The listing builds one solid part. Answer for the finished solid, in the listing's coordinates (mm). A direction names the side the tool comes from. Round coordinates to 2 decimals unless told otherwise and drop trailing zeros. Order: outer loops, then holes, each group sorted by start corner. A loop starts at its lowest first (then second) coordinate and runs counter-clockwise, first axis right, second up. Notation, with made-up numbers: (16.25, -28.5) - (60.25, -28.5) arc R23 ccw to (60.25, -19.5) - close; hole circle Ø2 at (-14.5, -4). An arc over 180 degrees is marked (long way). Write item = value, one per line.
from build123d import *

# Parameters (mm, degrees)
F0_R           = 31.75
F0_R_2         = 15.875
F1_DEPTH       = 50.8
F2_R           = 9.525
F3_DEPTH       = 31.75
F5_D           = 19.05
F5_CSINK_D     = 31.75
F5_CSINK_ANGLE = 82
F7_DEPTH       = 76.2


with BuildPart() as f1:
    # F0 (on Front) → F1 (new body)
    with BuildSketch(Plane.XZ):
        Circle(F0_R)
        Circle(F0_R_2, mode=Mode.SUBTRACT)
    extrude(amount=F1_DEPTH)

    # F2 (on Front) → F3 (join)
    with BuildSketch(Plane.XZ):
        with BuildLine():
            Line((76.2, 25.49937), (18.47559, 25.49937))
            Line((18.47559, 25.49937), (18.47559, -25.30063))
            Line((18.47559, -25.30063), (76.2, -25.30063))
            ThreePointArc((76.2, -25.30063), (101.6, 0.09937), (76.2, 25.49937))
        make_face()
        with Locations((76.2, 0)):
            Circle(F2_R, mode=Mode.SUBTRACT)
    extrude(amount=F3_DEPTH)

    # F5 (through all)
    with Locations(Plane.XZ.offset(31.75)):
        with Locations((76.2, 0.09937)):
            CounterSinkHole(F5_D / 2, F5_CSINK_D / 2, counter_sink_angle=F5_CSINK_ANGLE)

    # F6 (on face) → F7 (cut)
    with BuildSketch(Plane.XZ.offset(50.8)):
        with BuildLine():
            ThreePointArc((15.875, 0), (15.691131, -2.409153), (15.143785, -4.7625))
            Line((15.143785, -4.7625), (19.906285, -4.7625))
            Line((19.906285, -4.7625), (19.906285, 4.7625))
            Line((19.906285, 4.7625), (15.143785, 4.7625))
            ThreePointArc((15.143785, 4.7625), (15.691131, 2.409153), (15.875, 0))
        make_face()
    extrude(amount=-F7_DEPTH, mode=Mode.SUBTRACT)


solid = f1.part
Q1. Section A-A on x = 0 is taken. Determine the outline of the cut face in (y, z) (3 decimals).
Model answer:
outline = (-50.8, -31.75) - (0, -31.75) - (0, -15.875) - (-50.8, -15.875) - close; (-50.8, 15.875) - (0, 15.875) - (0, 31.75) - (-50.8, 31.75) - close
Q2. Determine the mould class of faces 4 (the face through (47, -16, -25.301)), 5 (the face through (101.594, -15.653, -0.459)), 6 (the face through (-15.862, -25.044, 0.63)) for opening direction Z: released by +Z, released by -Z, zero draft, split by the parting line, or undercut.
Model answer:
face_4 = released by -Z
face_5 = split by the parting line
face_6 = undercut
Q3. For faces 1 (the face through (34, 0, 0)), 2 (the face through (48, -16, 25.499)), 3 (the face through (75.99, -12.051, 9.622)), determine the directions among +Z, -Z, +X, -X, +Y, -Y from which every point of the face is accessible in a straight line to the end or side of a thin tool.
Model answer:
face_1 = +Z, -Z, +X, -X, +Y
face_2 = +Z, +X, +Y, -Y
face_3 = +Y, -Y
Q4. Section D-D on z = 18 is taken. Determine the outline of the cut face in (x, y).
Model answer:
outline = (-26.15, -50.8) - (26.15, -50.8) - (26.15, -31.75) - (94.22, -31.75) - (94.22, 0) - (-26.15, 0) - close
Q5. Flat-ended cylindrical pins translate along their axes: P1, Ø9.5, axis at x = 49.5, y = -15.5, coming from the +Z side; P2, Ø8, axis at x = 28, y = -7, coming from the -Z side; P3, Ø3, axis at x = -2, y = -7.5, coming from the -Z side. Find the tip coordinate at first contact, or state that the pin passes through.
Model answer:
P1 = 25.5
P2 = -25.3
P3 = -31.75
Q6. Find the intervals of material crossed by line 1 (X direction, y = -11, z = 0) (3 decimals); line 2 (Z direction, x = 0, y = -21) (3 decimals); line 3 (Y direction, x = 41, z = 16), in increasing order. Write a range as from..to.
Model answer:
line_1 = -31.75..-15.875, 19.906..66.675, 85.725..101.6
line_2 = -31.75..-15.875, 15.875..31.75
line_3 = -31.75..0
Q7. Section C-C on x = 33 is taken. Determine the outline of the cut face in (y, z), then the cut area to 3 significant figures.
Model answer:
outline = (-31.75, -25.3) - (0, -25.3) - (0, 25.5) - (-31.75, 25.5) - close
area = 1,610 mm^2
